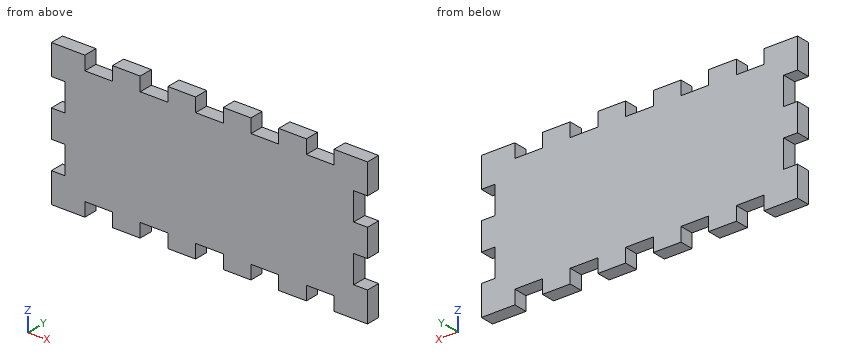
```python
from build123d import *

# Parameters (mm, degrees)
BOSS_EXTRUDE1_DEPTH = 6


with BuildPart() as part:
    # Sketch1 → Boss-Extrude1 (new body)
    with BuildSketch(Plane(origin=(0, 0, 0), x_dir=(1, 0, 0), z_dir=(0, 1, 0))):
        Polygon((-54, -31), (-54, -25), (-42, -25), (-42, -31), (-30, -31), (-30, -25), (-18, -25), (-18, -31), (-6, -31), (-6, -25), (6, -25), (6, -31), (18, -31), (18, -25), (30, -25), (30, -31), (42, -31), (42, -25), (54, -25), (54, -31), (66, -31), (68.499999877, -31), (68.499999877, -17.999998649), (66.000000123, -17.999998649), (62.500000123, -17.999998649), (62.500000123, -5.999998649), (66.000000123, -5.999998649), (68.499999877, -5.999998649), (68.499999877, 6), (66.000000123, 6), (62.500000123, 6), (62.500000123, 18), (66.000000123, 18), (68.499999877, 18), (68.499999877, 31), (66, 31), (54, 31), (54, 25), (42, 25), (42, 31), (30, 31), (30, 25), (18, 25), (18, 31), (6, 31), (6, 25), (-6, 25), (-6, 31), (-18, 31), (-18, 25), (-30, 25), (-30, 31), (-42, 31), (-42, 25), (-54, 25), (-54, 31), (-66, 31), (-68.499999877, 31), (-68.499999877, 18), (-66.000000123, 18), (-62.500000123, 18), (-62.500000123, 6), (-66.000000123, 6), (-68.499999877, 6), (-68.499999877, -5.999998649), (-66.000000123, -5.999998649), (-62.500000123, -5.999998649), (-62.500000123, -17.999998649), (-66.000000123, -17.999998649), (-68.499999877, -17.999998649), (-68.499999877, -31), (-66, -31), align=None)
    extrude(amount=BOSS_EXTRUDE1_DEPTH)


solid = part.part
```
Can you work these out from the model? Positions are in its coordinate system, mm. Coordinates: 2 decimals unless noted, no trailing zeros. Loops run counter-clockwise (first coordinate to the right, second up) from the corner with the lowest first, then second, coordinate; pieces in that order, holes last. Notation, with made-up numbers: (-4, 54) - (34, 54) arc R19 cw to (34, 73) - close; hole circle Ø1 at (26.25, 37.5). An arc over 180 degrees is marked (long way). Answer as CSV lines item,"result". Start each with the question number.
1) I need wall thicknesses on line 1 (X direction, y = 1.3, z = -26.5); line 2 (X direction, y = 0.5, z = -8); line 3 (Z direction, x = 46, y = 5.15). Which ranges of each line are inside material? Lowest first, please. Write a range as from..to.
2) For pin 1 (1.8 mm diameter, centred on y = 3.5, z = 9.5, fed in from +X); pin 2 (3 mm diameter, centred on x = -46, y = 3.5, fed in from -Z); pin 3 (1.8 mm diameter, centred on x = 48.5, y = 3.5, fed in from +Z), each with a flat end and sliding along its axis, tell me the tip position at first contact or that it passes through.
3) Suppose I cut it at B-B (x = 21). Please give me the cut outline in (y, z), plus the area to 3 significant figures.
4) Suppose I cut it at A-A (z = -13). Please give me the cut outline in (x, y).
Check result:
1,line 1,"x = -68.5..-54, -42..-30, -18..-6, 6..18, 30..42, 54..68.5"
1,line 2,"x = -62.5..62.5"
1,line 3,"z = -25..25"
2,pin 1,"stops at x = 62.5"
2,pin 2,"stops at z = -25"
2,pin 3,"stops at z = 25"
3,outline,"(0, -25) - (6, -25) - (6, 25) - (0, 25) - close"
3,area,"300 mm²"
4,outline,"(-62.5, 0) - (62.5, 0) - (62.5, 6) - (-62.5, 6) - close"
